```python
from build123d import *

# Parameters (mm, degrees)
F0_W           = 13.462
F0_H           = 13.462
F1_DEPTH       = 50.8
F5_D           = 5.1054
F5_DEPTH       = 22.86
F5_CBORE_D     = 25.5524
F5_CBORE_DEPTH = 11.0998
F5_TIP         = 1.5338169022
F6_D           = 17.4625
F6_DEPTH       = 23.8125
F6_TIP         = 5.2462642799


with BuildPart() as f1:
    # F0 (on Top) → F1 (new body)
    with BuildSketch(Plane.XY):
        with BuildLine():
            Line((-37.5396344488, 30.8131494279), (-17.9816344488, 30.8131494279))
            ThreePointArc((-17.9816344488, 30.8131494279), (-18.7067968135, 37.6952902366), (-20.8504328807, 44.2751494279))
            Line((-20.8504328807, 44.2751494279), (-51.0016344488, 44.2751494279))
            Line((-51.0016344488, 44.2751494279), (-51.0016344488, 30.8131494279))
            Line((-51.0016344488, 30.8131494279), (-37.5396344488, 30.8131494279))
        make_face()
        with BuildLine():
            Line((-51.0016344488, 44.2751494279), (-20.8504328807, 44.2751494279))
            ThreePointArc((-20.8504328807, 44.2751494279), (-51.0016344488, 63.8331494279), (-81.1528360169, 44.2751494279))
            Line((-81.1528360169, 44.2751494279), (-51.0016344488, 44.2751494279))
        make_face()
        with BuildLine():
            Line((-51.0016344488, 44.2751494279), (-81.1528360169, 44.2751494279))
            ThreePointArc((-81.1528360169, 44.2751494279), (-83.296472084, 37.6952902366), (-84.0216344488, 30.8131494279))
            Line((-84.0216344488, 30.8131494279), (-64.4636344488, 30.8131494279))
            Line((-64.4636344488, 30.8131494279), (-51.0016344488, 30.8131494279))
            Line((-51.0016344488, 30.8131494279), (-51.0016344488, 44.2751494279))
        make_face()
        with BuildLine():
            ThreePointArc((-84.0216344488, 30.8131494279), (-83.296472084, 23.9310086192), (-81.1528360169, 17.3511494279))
            Line((-81.1528360169, 17.3511494279), (-64.4636344488, 17.3511494279))
            Line((-64.4636344488, 17.3511494279), (-64.4636344488, 30.8131494279))
            Line((-64.4636344488, 30.8131494279), (-84.0216344488, 30.8131494279))
        make_face()
        with BuildLine():
            ThreePointArc((-81.1528360169, 17.3511494279), (-51.0016344488, -2.2068505721), (-20.8504328807, 17.3511494279))
            Line((-20.8504328807, 17.3511494279), (-37.5396344488, 17.3511494279))
            Line((-37.5396344488, 17.3511494279), (-51.0016344488, 17.3511494279))
            Line((-51.0016344488, 17.3511494279), (-64.4636344488, 17.3511494279))
            Line((-64.4636344488, 17.3511494279), (-81.1528360169, 17.3511494279))
        make_face()
        with BuildLine():
            ThreePointArc((-20.8504328807, 17.3511494279), (-18.7067968135, 23.9310086192), (-17.9816344488, 30.8131494279))
            Line((-17.9816344488, 30.8131494279), (-37.5396344488, 30.8131494279))
            Line((-37.5396344488, 30.8131494279), (-37.5396344488, 17.3511494279))
            Line((-37.5396344488, 17.3511494279), (-20.8504328807, 17.3511494279))
        make_face()
        with Locations((-57.7326344488, 24.0821494279)):
            Rectangle(F0_W, F0_H)
        with Locations((-44.2706344488, 24.0821494279)):
            Rectangle(F0_W, F0_H)
    extrude(amount=F1_DEPTH)

    # F5
    with Locations(Plane.XY.offset(50.8)):
        with Locations((-64.0826344488, 43.8941494279), (-37.9206344488, 43.8941494279), (-37.9206344488, 17.7321494279), (-64.0826344488, 17.7321494279)):
            CounterBoreHole(F5_D / 2, F5_CBORE_D / 2, F5_CBORE_DEPTH, depth=F5_DEPTH)
            with Locations((0, 0, -(F5_DEPTH + F5_TIP / 2))):  # 118° drill point
                Cone(0, F5_D / 2, F5_TIP, mode=Mode.SUBTRACT)

    # F6
    with Locations(Plane(origin=(0, 0, 0), x_dir=(1, 0, 0), z_dir=(0, 0, -1))):
        with Locations((-51.0016344488, -30.8131494279)):
            Hole(F6_D / 2, depth=F6_DEPTH)
            with Locations((0, 0, -(F6_DEPTH + F6_TIP / 2))):  # 118° drill point
                Cone(0, F6_D / 2, F6_TIP, mode=Mode.SUBTRACT)


solid = f1.part
```
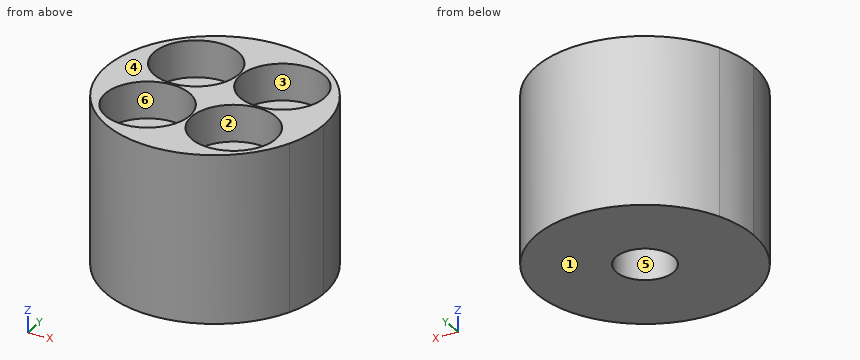
Verification items for the finished model (mm, model axes). Face numbers are marked on the shaded views. A direction names the side the tool comes from. Round coordinates to 2 decimals unless told otherwise and drop trailing zeros. Write each loop counter-clockwise with the first axis right and the second up, starting at its lowest first coordinate (ties: lowest second). Pieces come first, ordered by that corner, then holes.
1. Section check D-D on x = -68.5. Enter the section's corners in (y, z), plus the area to 3 significant figures.
2. Access from +Z, -Z, +X, -X, +Y, -Y to the whole of each face (thin tool, end or side, straight path). Record for the marked faces 4, 5 and 6.
3. Gauge pin test, flat ends, axial feed: P1, Ø1, axis at y = 37.5, z = 28.5, coming from the -X side; P2, Ø3, axis at y = 41.5, z = 32, coming from the +X side; P3, Ø7.5, axis at x = -63, y = 39, coming from the +Z side. Record the tip position at first contact, or that the pin passes through.
4. Section check B-B on y = 13. Enter the section's corners in (x, z), plus the area to 3 significant figures.
5. Section check A-A on z = 11.5. Enter the section's corners in (x, y), plus the area to 3 significant figures.
6. Scan lines: L1, parallel to X at y = 35.5, z = 44; L2, parallel to Y at x = -62, z = 48.5; L3, parallel to X at y = 50, z = 41.5. Record each from-to range of solid material in increasing order.
7. Draft check along X on the marked faces 1, 2 and 3. Enter one of: +X half, -X half, draft (parallel to the pull), parting line (faces both ways), or undercut.
8. Section check C-C on z = 44.5. Enter the section's corners in (x, y), plus the area to 3 significant figures.
Answer:
1. outline: (2.81, 0) - (58.82, 0) - (58.82, 50.8) - (55.88, 50.8) - (55.88, 39.7) - (31.91, 39.7) - (31.91, 50.8) - (29.72, 50.8) - (29.72, 39.7) - (5.74, 39.7) - (5.74, 50.8) - (2.81, 50.8) - close
1. area: 2,310 mm2
2. face 4: +Z, +X, -X, +Y, -Y
2. face 5: -Z
2. face 6: +Z
3. P1: stops at x = -83.44
3. P2: stops at x = -19.29
3. P3: stops at z = 39.7
4. outline: (-78.8, 0) - (-23.2, 0) - (-23.2, 50.8) - (-26.05, 50.8) - (-26.05, 39.7) - (-49.79, 39.7) - (-49.79, 50.8) - (-52.22, 50.8) - (-52.22, 39.7) - (-75.95, 39.7) - (-75.95, 50.8) - (-78.8, 50.8) - close
4. area: 2,300 mm2
5. outline: circle Ø66.04 at (-51, 30.81); hole circle Ø17.46 at (-51, 30.81)
5. area: 3,190 mm2
6. L1: x = -83.69 to -73.71, -54.45 to -47.55, -28.29 to -18.32
6. L2: y = -0.32 to 5.13, 30.34 to 31.29, 56.5 to 61.95
6. L3: x = -77.88 to -75.31, -52.86 to -49.14, -26.7 to -24.13
7. face 1: draft
7. face 2: undercut
7. face 3: undercut
8. outline: circle Ø66.04 at (-51, 30.81); hole circle Ø25.55 at (-64.08, 17.73); hole circle Ø25.55 at (-64.08, 43.89); hole circle Ø25.55 at (-37.92, 17.73); hole circle Ø25.55 at (-37.92, 43.89)
8. area: 1,370 mm2
